Model file for the job. Use its own axes, mm. Face numbers are marked on the shaded views. Round coordinates to 2 decimals unless told otherwise and drop trailing zeros. Order: outer loops, then holes, each group sorted by start corner. A loop starts at its lowest first (then second) coordinate and runs counter-clockwise, first axis right, second up. Notation, with made-up numbers: (57.5, -2) - (116.5, -2) arc R23 ccw to (116.5, 17) - close; hole circle Ø6 at (6, 24.25). An arc over 180 degrees is marked (long way). Write item = value, one per line. Start each with the question number.
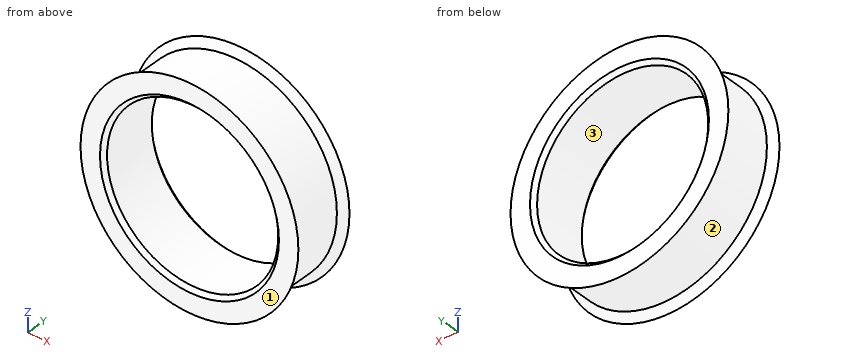
from build123d import *

# Parameters (mm, degrees)
SKETCH001_R  = 11
POCKET_DEPTH = 8
CHAMFER_SIZE = 0.5


with BuildPart() as part:
    # Sketch → Revolution (revolve)
    with BuildSketch(Plane.XY):
        Polygon((0, 0), (-14, 0), (-13, 0.75), (-13, 7.25), (-14, 8), (0, 8), align=None)
    revolve(axis=Axis((0, 0, 0), (0, 1, 0)))

    # Sketch001 (on Face1 of Revolution) → Pocket (cut)
    with BuildSketch(Plane.XZ):
        Circle(SKETCH001_R)
    extrude(amount=-POCKET_DEPTH, mode=Mode.SUBTRACT)

    # Chamfer
    chamfer_edges = [part.edges().sort_by_distance(p)[0] for p in [
        (-11, 0, 0),
        (-11, 8, 0),
    ]]
    chamfer(chamfer_edges, length=CHAMFER_SIZE)


solid = part.part
Item 1: Saw through at C-C, the plane y = 6.5. Give the cut face in (x, z), then the cut area to 3 significant figures.
Item 2: Mould opens along Z. For the marked faces 1, 2 and 3 say: +Z half, -Z half, draft (parallel to the pull), parting line (faces both ways), or undercut.
Item 3: Saw through at B-B, the plane z = 0. Give the cut face in (x, y), then the cut area to 3 significant figures.
Item 4: Probe L1, parallel to Z at x = 0, y = 4.75; L2, parallel to X at y = 3.5, z = -5.5; L3, parallel to Z at x = 8, y = 2.25. List the from-to ranges inside material, lowest first.
Item 5: Saw through at A-A, the plane x = 0. Give the cut face in (y, z), then the cut area to 3 significant figures.
Item 6: Drop flat-ended pins along their axis: pin 1 (4 mm diameter, centred on y = 3.5, z = -4, fed in from +X); pin 2 (5 mm diameter, centred on x = 7.5, z = 1, fed in from +Y). Give the stop position or say it passes through.
Check sheet entries:
q1.outline = circle Ø26 at (0, 0); hole circle Ø22 at (0, 0)
q1.area = 151 mm2
q2.face_1 = draft
q2.face_2 = parting line
q2.face_3 = undercut
q3.outline = (-14, 0) - (-11.5, 0) - (-11, 0.5) - (-11, 7.5) - (-11.5, 8) - (-14, 8) - (-13, 7.25) - (-13, 0.75) - close; (11, 0.5) - (11.5, 0) - (14, 0) - (13, 0.75) - (13, 7.25) - (14, 8) - (11.5, 8) - (11, 7.5) - close
q3.area = 33.0 mm2
q4.L1 = -13 to -11, 11 to 13
q4.L2 = -11.78 to -9.53, 9.53 to 11.78
q4.L3 = -10.25 to -7.55, 7.55 to 10.25
q5.outline = (0, -14) - (0.75, -13) - (7.25, -13) - (8, -14) - (8, -11.5) - (7.5, -11) - (0.5, -11) - (0, -11.5) - close; (0, 11.5) - (0.5, 11) - (7.5, 11) - (8, 11.5) - (8, 14) - (7.25, 13) - (0.75, 13) - (0, 14) - close
q5.area = 33.0 mm2
q6.pin_1 = 12.85
q6.pin_2 = through
